Answer from the drawing. Dimensions are ordinates in mm from the lowest x, y and z of the part. A direction names the side the tool comes from. Coordinates: 2 decimals unless noted, no trailing zeros. Order: outer loops, then holes, each group sorted by start corner. A loop starts at its lowest first (then second) coordinate and runs counter-clockwise, first axis right, second up. Notation, with made-up numbers: M 84.25,39 L 121.25,39 A21 cw 121.25,72 Z; hole C 75.5,75 d6. An arc over 180 degrees is marked long. Use a Markdown table: item, result.
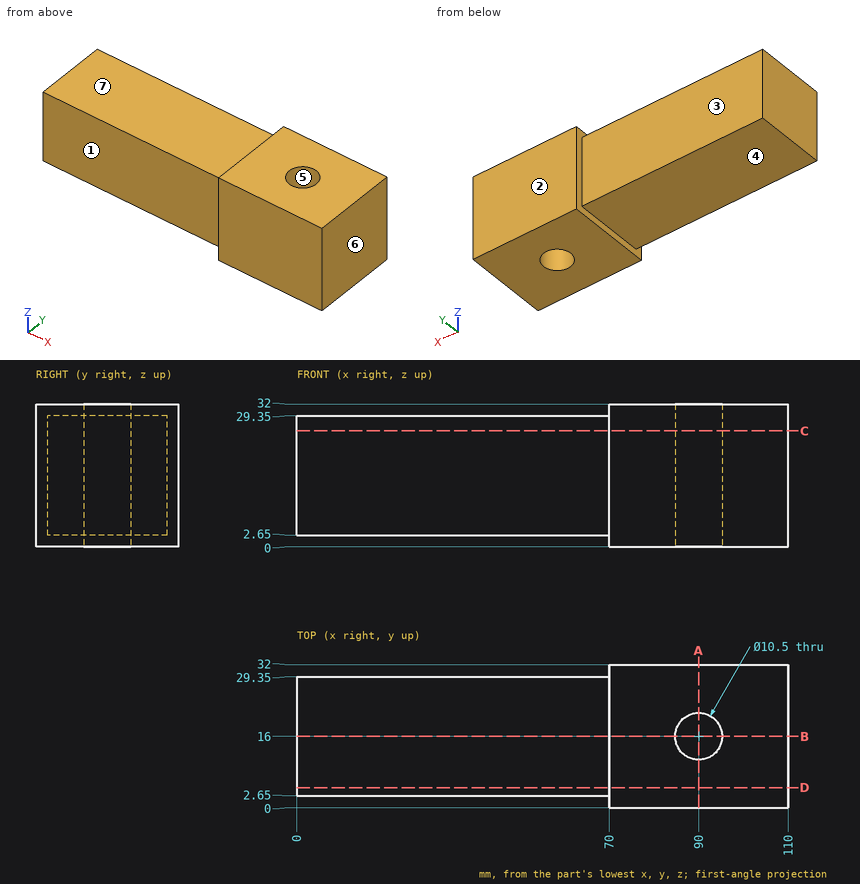
(1) A cutting plane is placed at C-C (z = 26). Determine the outline of the cut face in (x, y), then the cut area to 3 significant figures.
Conclusion:
| item | result |
|---|---|
| outline | M 0,2.65 L 70,2.65 L 70,0 L 110,0 L 110,32 L 70,32 L 70,29.35 L 0,29.35 Z; hole C 90,16 d10.5 |
| area | 3,060 mm2 |
(2) Straight lines are drawn through the part: L1, parallel to X at y = 25, z = 2; L2, parallel to Z at x = 8, y = 22. For each, find the intervals that lie inside material, in ascending order.
Conclusion:
| item | result |
|---|---|
| L1 | 70 to 110 |
| L2 | 2.65 to 29.35 |
(3) A cutting plane is placed at A-A (x = 90). Determine the outline of the cut face in (y, z), then the cut area to 3 significant figures.
Conclusion:
| item | result |
|---|---|
| outline | M 0,0 L 10.75,0 L 10.75,32 L 0,32 Z; M 21.25,0 L 32,0 L 32,32 L 21.25,32 Z |
| area | 688 mm2 |
(4) A cutting plane is placed at D-D (y = 4.5). Determine the outline of the cut face in (x, z).
Conclusion:
| item | result |
|---|---|
| outline | M 0,2.65 L 70,2.65 L 70,0 L 110,0 L 110,32 L 70,32 L 70,29.35 L 0,29.35 Z |
(5) A cutting plane is placed at B-B (y = 16). Determine the outline of the cut face in (x, z).
Conclusion:
| item | result |
|---|---|
| outline | M 0,2.65 L 70,2.65 L 70,0 L 84.75,0 L 84.75,32 L 70,32 L 70,29.35 L 0,29.35 Z; M 95.25,0 L 110,0 L 110,32 L 95.25,32 Z |
(6) Given P1, Ø1.5, axis at x = 46, y = 25.5, coming from the -Z side; P2, Ø8.5, axis at x = 90, y = 16, coming from the +Z side; P3, Ø1, axis at x = 46, z = 10.5, coming from the -Y side; P4, Ø3, axis at x = 11, z = 11.5, coming from the +Y side, each flat-ended and moving along its own axis, determine where each tip first touches the part or whether it passes through.
Conclusion:
| item | result |
|---|---|
| P1 | z = 2.65 |
| P2 | through |
| P3 | y = 2.65 |
| P4 | y = 29.35 |
(7) Determine the mould class of the marked faces 5, 6 and 7 for opening direction X: pulls with the +X half, pulls with the -X half, needs draft (parallel to the pull), parting line crosses it, or undercut.
Conclusion:
| item | result |
|---|---|
| face 5 | undercut |
| face 6 | pulls with the +X half |
| face 7 | needs draft |
(8) Which of the six approach directions +Z, -Z, +X, -X, +Y, -Y give full straight-line access (tool end or side, diameter ignored) to the marked faces 1, 2, 3 and 4?
Conclusion:
| item | result |
|---|---|
| face 1 | +Z, -Z, -X, -Y |
| face 2 | +Z, -Z, +X, -X, +Y |
| face 3 | +Z, -Z, -X, +Y |
| face 4 | -Z, -X, +Y, -Y |
